Model file for the job. Use its own axes, mm. A direction names the side the tool comes from. Give positions to 0.01 mm unless a question says otherwise; leave off trailing zeros. Write each loop counter-clockwise with the first axis right and the second up, starting at its lowest first coordinate (ties: lowest second). Pieces come first, ordered by that corner, then holes.
```python
from build123d import *

# Parameters (mm, degrees)
F1_DEPTH  = 20
F2_W      = 30.5
F2_H      = 10
F3_DEPTH  = 30
F4_W      = 30.5
F4_H      = 10
F5_DEPTH  = 30
F7_DEPTH  = 47.5
F8_W      = 10
F8_H      = 20
F8_H_2    = 10
F9_DEPTH  = 20
F10_W     = 10
F10_H     = 10
F11_DEPTH = 10
F13_DEPTH = 150


with BuildPart() as f1:
    # F0 (on Front) → F1 (new body)
    with BuildSketch(Plane.XZ):
        Polygon((-10, 0), (0, 0), (0, 100), (-10, 100), (-10, 50), (-57.5, 50), (-57.5, 20), (-10, 20), align=None)
        Polygon((0, 100), (0, 0), (10, 0), (10, 20), (57.5, 20), (57.5, 50), (10, 50), (10, 100), align=None)
    extrude(amount=F1_DEPTH)

    # F2 (on face) → F3 (cut, through all)
    with BuildSketch(Plane(origin=(0, 0, 20), x_dir=(1, 0, 0), z_dir=(0, 0, -1))):
        with Locations((-42.25, 15)):
            Rectangle(F2_W, F2_H)
    extrude(amount=-F3_DEPTH, mode=Mode.SUBTRACT)

    # F4 (on face) → F5 (cut, through all)
    with BuildSketch(Plane(origin=(0, 0, 20), x_dir=(1, 0, 0), z_dir=(0, 0, -1))):
        with Locations((42.25, 15)):
            Rectangle(F4_W, F4_H)
    extrude(amount=-F5_DEPTH, mode=Mode.SUBTRACT)

    # F6 (on face) → F7 (cut, through all)
    with BuildSketch(Plane(origin=(-57.5, 0, 0), x_dir=(0, -1, 0), z_dir=(-1, 0, 0))):
        Polygon((0, 28), (0, 20), (4, 20), (4, 28), (0, 31), align=None)
    extrude(amount=-F7_DEPTH, mode=Mode.SUBTRACT)

    # F8 (on face) → F9 (cut, through all)
    with BuildSketch(Plane.XZ.offset(20)):
        with Locations((0, 80)):
            Rectangle(F8_W, F8_H)
        with Locations((0, 40)):
            Rectangle(F8_W, F8_H)
        with Locations((0, 5)):
            Rectangle(F8_W, F8_H_2)
    extrude(amount=-F9_DEPTH, mode=Mode.SUBTRACT)

    # F10 (on face) → F11 (cut)
    with BuildSketch(Plane(origin=(0, 0, 0), x_dir=(-1, 0, 0), z_dir=(0, 1, 0))):
        with Locations((0, 65)):
            Rectangle(F10_W, F10_H)
        with Locations((0, 25)):
            Rectangle(F10_W, F10_H)
    extrude(amount=-F11_DEPTH, mode=Mode.SUBTRACT)

    # F12 (on face) → F13 (cut)
    with BuildSketch(Plane.YZ.offset(57.5)):
        Polygon((-4, 20), (0, 20), (0, 28), (0, 31), (-4, 28), align=None)
    extrude(amount=-F13_DEPTH, mode=Mode.SUBTRACT)


solid = f1.part
```
1. Probe probe 1 along Z at (x, y) = (-1.5, -11.75); probe 2 along X at (y, z) = (-2.25, 39.5); probe 3 along X at (y, z) = (-1.25, 61.5). List the from-to ranges inside material, lowest first.
Calculated:
probe 1: z = 10 to 30, 50 to 70, 90 to 100
probe 2: x = -57.5 to -5, 5 to 57.5
probe 3: x = -10 to -5, 5 to 10
2. Slice it at B-B, the plane y = -8.75. Write the cut outline in (x, z).
Calculated:
outline: (-57.5, 20) - (-10, 20) - (-10, 0) - (-5, 0) - (-5, 10) - (5, 10) - (5, 0) - (10, 0) - (10, 20) - (57.5, 20) - (57.5, 50) - (10, 50) - (10, 100) - (-10, 100) - (-10, 50) - (-57.5, 50) - close; hole (-5, 20) - (5, 20) - (5, 50) - (-5, 50) - close; hole (-5, 60) - (5, 60) - (5, 90) - (-5, 90) - close
3. Slice it at C-C, the plane z = 24.5. Write the cut outline in (x, y), and give its area (3 significant figures).
Calculated:
outline: (-57.5, -10) - (-27, -10) - (-27, -20) - (27, -20) - (27, -10) - (57.5, -10) - (57.5, -4) - (5, -4) - (5, -10) - (-5, -10) - (-5, -4) - (-57.5, -4) - close
area: 1,170 mm2
4. Slice it at A-A, the plane z = 40. Write the cut outline in (x, y), and give its area (3 significant figures).
Calculated:
outline: (-57.5, -10) - (-27, -10) - (-27, -20) - (-5, -20) - (-5, 0) - (-57.5, 0) - close; (5, -20) - (27, -20) - (27, -10) - (57.5, -10) - (57.5, 0) - (5, 0) - close
area: 1,490 mm2
5. Which spindle directions (+Z, -Z, +X, -X, +Y, -Y) get a long thin tool onto all of the face, cutting with end or side? Do faces 4 (the flat face through (-10, -10, 10)), 5 (the flat face through (0, -15, 70)), 6 (the flat face through (-5, -10, 78)), 7 (the flat face through (5, -10, 5)). Say none if no direction does.
Calculated:
face 4: -Z, -X, +Y, -Y
face 5: +Y, -Y
face 6: +Y
face 7: -Z, +Y, -Y
6. Slice it at D-D, the plane x = -7.5. Write the cut outline in (y, z), and give its area (3 significant figures).
Calculated:
outline: (-20, 0) - (0, 0) - (0, 20) - (-4, 20) - (-4, 28) - (0, 31) - (0, 100) - (-20, 100) - close
area: 1,960 mm2
7. Pin check, flat tips, straight feed: P1, Ø8, axis at y = -14.5, z = 89.5, coming from the -X side; P2, Ø5, axis at x = -30, y = -10, coming from the -Z side; P3, Ø4, axis at x = -31.5, z = 24.5, coming from the +Y side. Stop position of each tip, or through.
Calculated:
P1: stops at x = -10
P2: stops at z = 20
P3: stops at y = -4
8. Pull direction X, two halves, no side cores. Call faces 1 (the flat face through (7, -10, 0)), 2 (the flat face through (-10, -10, 75)), 3 (the flat face through (0, -10, 65)): +X half, -X half, draft (parallel to the pull), parting line (faces both ways), or undercut.
Calculated:
face 1: draft
face 2: -X half
face 3: undercut
